Part print with two shaded views. Sizes in mm from the minimum x, y, z corner. A direction names the side the tool comes from. Round coordinates to 2 decimals unless told otherwise and drop trailing zeros. Order: outer loops, then holes, each group sorted by start corner. A loop starts at its lowest first (then second) coordinate and runs counter-clockwise, first axis right, second up. Notation, with made-up numbers: (71, -3.75) -> (79, -3.75) arc R16 ccw to (79, 8.25) -> close; hole circle Ø2 at (-28, -36.5). An arc over 180 degrees is marked (long way). Answer as a JSON object with one key per item and string values.
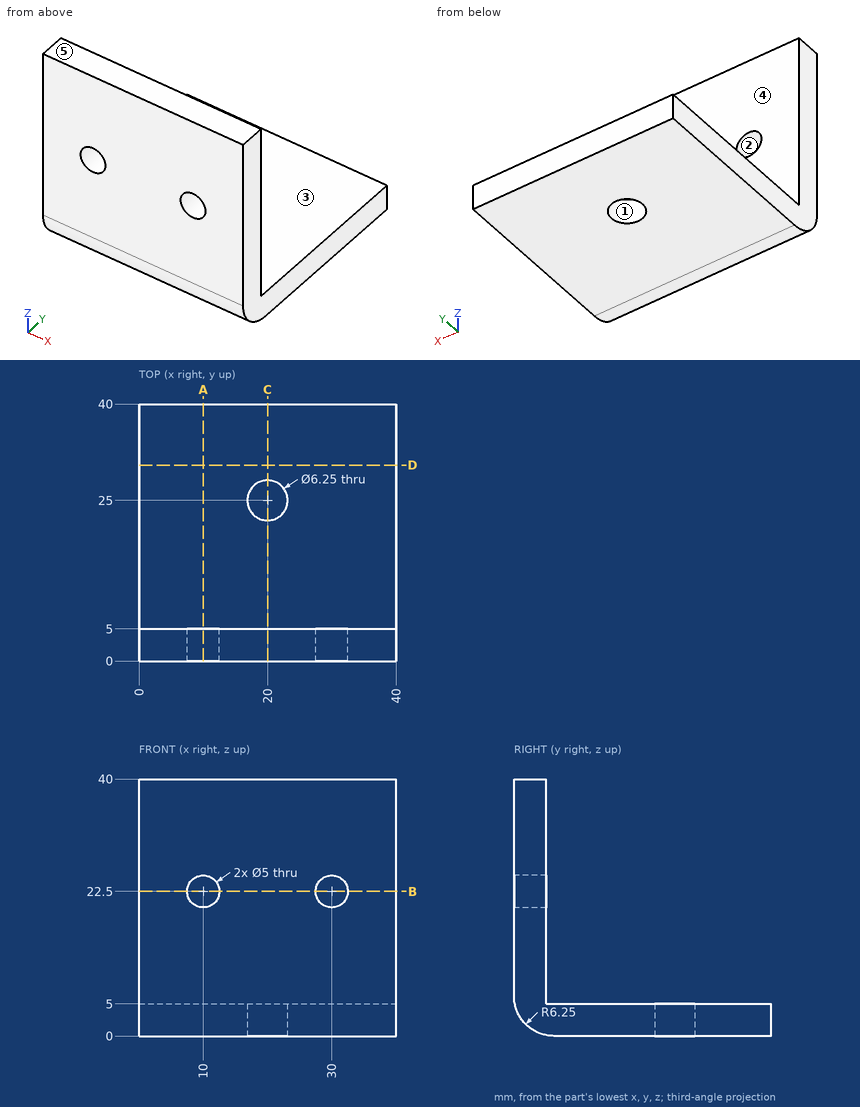
1) Cut at B-B, the plane z = 22.5. Give the cut face in (x, y).
Checked values:
{"outline": "(0, 0) -> (7.5, 0) -> (7.5, 5) -> (0, 5) -> close; (12.5, 0) -> (27.5, 0) -> (27.5, 5) -> (12.5, 5) -> close; (32.5, 0) -> (40, 0) -> (40, 5) -> (32.5, 5) -> close"}
2) Flat gauge pins, fed straight in: pin 1 Ø6 at (x, z) = (10, 22.5) entering from +Y; pin 2 Ø10.5 at (x, y) = (19, 18) entering from +Z. Where does each tip first touch, or does it go through?
Checked values:
{"pin 1": "stops at y = 5", "pin 2": "stops at z = 5"}
3) Cut at C-C, the plane x = 20. Give the cut face in (y, z) (3 decimals).
Checked values:
{"outline": "(0, 6.25) arc R6.25 ccw to (6.25, 0) -> (21.875, 0) -> (21.875, 5) -> (5, 5) -> (5, 40) -> (0, 40) -> close; (28.125, 0) -> (40, 0) -> (40, 5) -> (28.125, 5) -> close"}
4) Pull direction Z, two halves, no side cores. Call the marked faces 1, 2 and 3: pulls with the +Z half, pulls with the -Z half, needs draft (parallel to the pull), parting line crosses it, or undercut.
Checked values:
{"face 1": "needs draft", "face 2": "undercut", "face 3": "pulls with the +Z half"}
5) Cut at D-D, the plane y = 30.5. Give the cut face in (x, z).
Checked values:
{"outline": "(0, 0) -> (40, 0) -> (40, 5) -> (0, 5) -> close"}
6) Probe L1, parallel to X at y = 2.35, z = 22.5; L2, parallel to Y at x = 25.5, z = 14.5; L3, parallel to X at y = 1, z = 22. List the from-to ranges inside material, lowest first. Write a range as from..to.
Checked values:
{"L1": "x = 0..7.5, 12.5..27.5, 32.5..40", "L2": "y = 0..5", "L3": "x = 0..7.55, 12.45..27.55, 32.45..40"}
7) Which spindle directions (+Z, -Z, +X, -X, +Y, -Y) get a long thin tool onto all of the face, cutting with end or side? Do the marked faces 4 and 5. Say none if no direction does.
Checked values:
{"face 4": "+Z, +X, -X, +Y", "face 5": "+Z, +X, -X, +Y, -Y"}
8) Cut at A-A, the plane x = 10. Give the cut face in (y, z), plus the area to 3 significant figures.
Checked values:
{"outline": "(0, 6.25) arc R6.25 ccw to (6.25, 0) -> (40, 0) -> (40, 5) -> (5, 5) -> (5, 20) -> (0, 20) -> close; (0, 25) -> (5, 25) -> (5, 40) -> (0, 40) -> close", "area": "342 mm²"}
